For this review, take the finished solid that the model builds, in its own axes (mm). Coordinates: 2 decimals unless noted, no trailing zeros. Loops run counter-clockwise (first coordinate to the right, second up) from the corner with the lowest first, then second, coordinate; pieces in that order, holes last. Notation, with made-up numbers: (-8, 50) - (2, 50) arc R23 ccw to (2, 72) - close; hole circle Ø4 at (18.25, -11.75). An arc over 180 degrees is marked (long way). Answer as a JSON object with one key per item and string values. Group by question number.
Item 1: To check wall thickness, follow line 1 (Y direction, x = 78, z = 1.05); line 2 (Y direction, x = 145.35, z = 2.2). State the ranges of each line that lie inside material, in increasing order.
Item 2: Clearance check with a flat-ended pin moving along its axis: pin 1 (1 mm diameter, centred on x = 63.5, z = 1.5, fed in from +Y). State where the tip first meets the part, or that it passes through.
Item 3: We need section B-B (z = 0.85). State how many separate pieces and enclosed holes the cut face has, then the cut area to 3 significant figures.
Item 4: We need section A-A (x = 105). Give the boundary of the cut face in (y, z).
Item 5: We need section C-C (x = 62.5). Give the boundary of the cut face in (y, z), then the cut area to 3 significant figures.
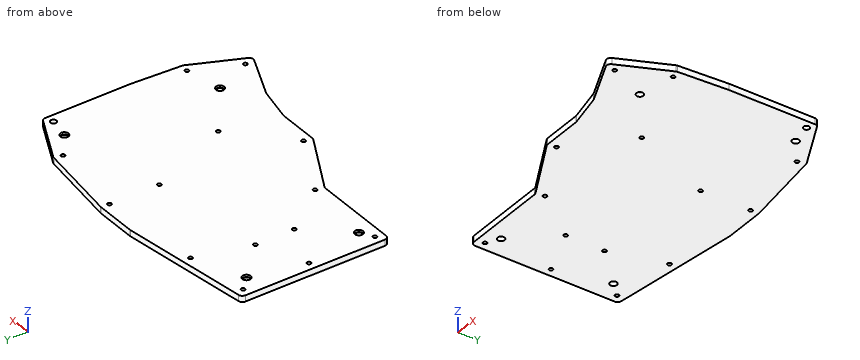
from build123d import *

# Parameters (mm, degrees)
PAD001_DEPTH    = 3
FILLET001_R     = 2
SKETCH016_R     = 0.95
SKETCH016_R_2   = 1.45
POCKET006_DEPTH = 3.001
SKETCH017_R     = 1.7
POCKET007_DEPTH = 3.001
SKETCH018_R     = 2
POCKET008_DEPTH = 1.1


with BuildPart() as part:
    # Sketch001 → Pad001 (new body)
    with BuildSketch(Plane.XY):
        Polygon((0, 0), (0, 72.168726), (64.627307, 80.65), (84.722693, 80.65), (124.674612, 75.406966), (149.35, 63.069272), (149.35, 19.79532), (147.938038, -4.774436), (136.341223, -30.821308), (112.397959, -20.161079), (95.409166, -16.55), (75.203903, -16.55), (44.103903, 0), align=None)
    extrude(amount=PAD001_DEPTH)

    # Fillet001
    fillet001_edges = [part.edges().sort_by_distance(p)[0] for p in [
        (0, 0, 1.5),
        (44.103903, 0, 1.5),
        (75.203903, -16.55, 1.5),
        (95.409166, -16.55, 1.5),
        (112.397959, -20.161079, 1.5),
        (136.341223, -30.821308, 1.5),
        (147.938038, -4.774436, 1.5),
        (149.35, 19.79532, 1.5),
        (149.35, 63.069272, 1.5),
        (124.674612, 75.406966, 1.5),
        (84.722693, 80.65, 1.5),
        (64.627307, 80.65, 1.5),
        (0, 72.168726, 1.5),
    ]]
    fillet(fillet001_edges, radius=FILLET001_R)

    # Sketch016 (on Face5 of Fillet001) → Pocket006 (cut, through all)
    with BuildSketch(Plane.XY.offset(3)):
        with Locations((4, 68.659363)):
            Circle(SKETCH016_R)
        with Locations((4, 36.329682)):
            Circle(SKETCH016_R)
        with Locations((4, 4)):
            Circle(SKETCH016_R)
        with Locations((45.101951, 4)):
            Circle(SKETCH016_R)
        with Locations((76.201951, -12.55)):
            Circle(SKETCH016_R)
        with Locations((134.313988, -25.540179)):
            Circle(SKETCH016_R)
        with Locations((143.986562, -3.815223)):
            Circle(SKETCH016_R)
        with Locations((145.35, 60.597136)):
            Circle(SKETCH016_R_2)
        with Locations((123.487306, 71.528483)):
            Circle(SKETCH016_R)
        with Locations((84.198914, 52.349499)):
            Circle(SKETCH016_R)
        with Locations((27.061811, 46.097252)):
            Circle(SKETCH016_R)
        with Locations((27.055561, 27.04681)):
            Circle(SKETCH016_R)
        with Locations((101.461166, 11.216918)):
            Circle(SKETCH016_R)
        with Locations((34.444327, 72.654682)):
            Circle(SKETCH016_R)
        with Locations((84.461347, 76.65)):
            Circle(SKETCH016_R)
    extrude(amount=-POCKET006_DEPTH, mode=Mode.SUBTRACT)

    # Sketch017 (on Face5 of Pocket006) → Pocket007 (cut, through all)
    with BuildSketch(Plane.XY.offset(3)):
        with Locations((10.086737, 62.606358)):
            Circle(SKETCH017_R)
        with Locations((10.086737, 7.515739)):
            Circle(SKETCH017_R)
        with Locations((126.131942, -7.312394)):
            Circle(SKETCH017_R)
        with Locations((135.066086, 62.606358)):
            Circle(SKETCH017_R)
    extrude(amount=-POCKET007_DEPTH, mode=Mode.SUBTRACT)

    # Sketch018 (on Face5 of Pocket007) → Pocket008 (cut)
    with BuildSketch(Plane.XY.offset(3)):
        with Locations((10.086737, 62.606358)):
            Circle(SKETCH018_R)
        with Locations((10.086737, 7.515739)):
            Circle(SKETCH018_R)
        with Locations((126.131942, -7.312394)):
            Circle(SKETCH018_R)
        with Locations((135.066086, 62.606358)):
            Circle(SKETCH018_R)
    extrude(amount=-POCKET008_DEPTH, mode=Mode.SUBTRACT)


solid = part.part
Check sheet entries:
{
 "1": {"line 1": "y = -16.55 to 80.65", "line 2": "y = -10.59 to 59.15, 62.05 to 65.07"},
 "2": {"pin 1": "stops at y = 80.57"},
 "3": {"separate pieces": "1", "enclosed holes": "19", "area": "13,000 mm2"},
 "4": {"outline": "(-18.59, 0) - (77.99, 0) - (77.99, 3) - (-18.59, 3) - close"},
 "5": {"outline": "(-9.79, 0) - (80.37, 0) - (80.37, 3) - (-9.79, 3) - close", "area": "270 mm2"}
}
